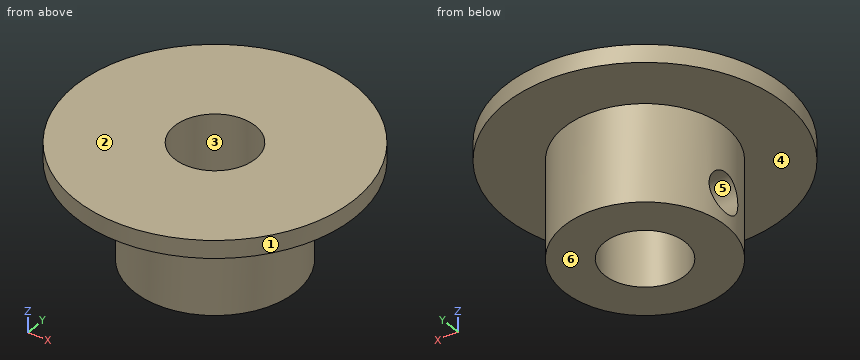
Autodesk Inventor part; units mm, degrees
ref_plane "YZ Plane" through (0, 0, 0) normal (1, 0, 0) x (0, 1, 0)
ref_plane "XZ Plane" through (0, 0, 0) normal (0, 1, 0) x (-1, 0, 0)
ref_plane "XY Plane" through (0, 0, 0) normal (0, 0, 1) x (1, 0, 0)
sketch "Sketch1" plane through (0, 0, 0) normal (0, 0, 1) x (1, 0, 0)
  line L0 (0, 7) -> (0, -7)
  line L1 (-7, 0) -> (7, 0)
  circle A0 centre (0, 0) radius 5
  circle A1 centre (0, 0) radius 2.5
  dimension "d0" = 10
  dimension "d1" = 5
extrude "Extrusion1" add sketch "Sketch1" along normal blind 6 contours A0 L1 A1 L0 | L0 A1 L1 A0 | A0 L0 A1 L1 | L1 A1 L0 A0
sketch "Sketch2" plane through (0, 0, 6) normal (0, 0, 1) x (1, 0, 0)
  circle A0 centre (0, 0) radius 2.5
  circle A1 centre (0, 0) radius 5
  circle A2 centre (0, 0) radius 8.625
  dimension "d4" = 17.25
extrude "Extrusion2" add sketch "Sketch2" along normal blind 1.1 contours A1 | A2
sketch "Sketch3" plane through (0, 0, 0) normal (1, 0, 0) x (0, 1, 0)
  line L0 (0, 8.52) -> (0, -1.42)
  line L1 (-12.075, 0) -> (12.075, 0)
  point P0 (0, 0)
  point P1 (0, 2)
  dimension "d7" = 2
hole "Hole1" at (0, 0, 2) direction (-1, 0, 0) diameter 2.4638 end through all
For this review, take the finished solid that the model builds, in its own axes (mm). Face numbers are marked on the shaded views. A direction names the side the tool comes from. Round coordinates to 2 decimals unless told otherwise and drop trailing zeros. Loops run counter-clockwise (first coordinate to the right, second up) from the corner with the lowest first, then second, coordinate; pieces in that order, holes last. Notation, with made-up numbers: (-5, 54) - (5, 54) arc R23 cw to (5, 87) - close; hole circle Ø4 at (37.25, 40). An arc over 180 degrees is marked (long way). One line per item, written item: value. Start each with the question number.
Item 1: Take a section at C-C (y = -1.75). Give the boundary of the cut face in (x, z), plus the area to 3 significant figures.
Item 2: For L1, parallel to X at y = 2.25, z = 4; L2, parallel to Z at x = 2.5, y = 5.5; L3, parallel to Y at x = 0, z = 4.25, list the stretches that pass through material, from the lowest coordinate up.
Item 3: For the marked faces 4, 5 and 6, list the 3-axis set-ups (+Z, -Z, +X, -X, +Y, -Y) from which the entire face can be reached by the end or side of a thin tool; tool diameter is ignored.
Item 4: Take a section at D-D (z = 5.5). Give the boundary of the cut face in (x, y), plus the area to 3 significant figures.
Item 5: Take a section at B-B (x = 0). Give the boundary of the cut face in (y, z) (3 decimals).
Item 6: Take a section at A-A (y = 0). Give the boundary of the cut face in (x, z) (3 decimals).
Item 7: Clearance check with flat-ended pins moving along their axes: pin 1 Ø3 at (y, z) = (0, 2) entering from -X; pin 2 Ø1 at (x, z) = (2, 6.5) entering from -Y; pin 3 Ø1 at (x, z) = (1.5, 1) entering from -Y. State where each tip first meets the part, or that it passes through.
Item 8: The part is to be moulded in two halves that separate along X. For the marked faces 1, 2 and 3, say which applies: +X half, -X half, draft (parallel to the pull), parting line (faces both ways), or undercut.
Answer below:
1. outline: (-8.45, 6) - (-4.68, 6) - (-4.68, 0) - (-1.79, 0) - (-1.79, 7.1) - (-8.45, 7.1) - close; (1.79, 0) - (4.68, 0) - (4.68, 6) - (8.45, 6) - (8.45, 7.1) - (1.79, 7.1) - close
1. area: 49.4 mm2
2. L1: x = -4.47 to -1.09, 1.09 to 4.47
2. L2: z = 6 to 7.1
2. L3: y = -5 to -2.5, 2.5 to 5
3. face 4: -Z
3. face 5: -X
3. face 6: -Z, +X, -X, +Y, -Y
4. outline: circle Ø10 at (0, 0); hole circle Ø5 at (0, 0)
4. area: 58.9 mm2
5. outline: (-8.625, 6) - (-5, 6) - (-5, 0) - (-2.5, 0) - (-2.5, 7.1) - (-8.625, 7.1) - close; (2.5, 0) - (5, 0) - (5, 6) - (8.625, 6) - (8.625, 7.1) - (2.5, 7.1) - close
6. outline: (-8.625, 6) - (-5, 6) - (-5, 3.232) - (-2.5, 3.232) - (-2.5, 7.1) - (-8.625, 7.1) - close; (-5, 0) - (-2.5, 0) - (-2.5, 0.768) - (-5, 0.768) - close; (2.5, 0) - (5, 0) - (5, 6) - (8.625, 6) - (8.625, 7.1) - (2.5, 7.1) - close
7. pin 1: stops at x = -5
7. pin 2: stops at y = -8.49
7. pin 3: stops at y = -4.9
8. face 1: parting line
8. face 2: draft
8. face 3: undercut
